from build123d import *

# Parameters (mm, degrees)
SKETCH1_W           = 137
SKETCH1_H           = 60
BOSS_EXTRUDE1_DEPTH = 6.5
SKETCH2_W           = 101
SKETCH2_H           = 55.5
CUT_EXTRUDE1_DEPTH  = 1.65
SKETCH3_W           = 87.3
SKETCH3_H           = 55.5
CUT_EXTRUDE2_DEPTH  = 4.1
SKETCH4_W           = 75.4
SKETCH4_H           = 51.7
CUT_EXTRUDE3_DEPTH  = 1.75
FILLET1_R           = 1
SKETCH6_W           = 7.15
SKETCH6_H           = 8
SKETCH6_W_2         = 6.55
CUT_EXTRUDE4_DEPTH  = 2.5
FILLET2_R           = 3
CHAMFER1_SIZE       = 0.5
SKETCH7_W           = 21
SKETCH7_H           = 52.453625608
CUT_EXTRUDE5_DEPTH  = 7.5
FILLET3_R           = 3
FILLET5_R           = 2
CHAMFER3_SIZE       = 1
FILLET6_R           = 1.5
FILLET7_R           = 1


with BuildPart() as part:
    # Sketch1 → Boss-Extrude1 (new body)
    with BuildSketch(Plane(origin=(0, 0, 0), x_dir=(1, 0, 0), z_dir=(0, 1, 0))):
        Rectangle(SKETCH1_W, SKETCH1_H)
    extrude(amount=BOSS_EXTRUDE1_DEPTH)

    # Sketch2 → Cut-Extrude1 (cut)
    with BuildSketch(Plane(origin=(0, 6.5, 0), x_dir=(1, 0, 0), z_dir=(0, 1, 0))):
        with Locations((14, 0)):
            Rectangle(SKETCH2_W, SKETCH2_H)
    extrude(amount=-CUT_EXTRUDE1_DEPTH, mode=Mode.SUBTRACT)

    # Sketch3 → Cut-Extrude2 (cut)
    with BuildSketch(Plane(origin=(0, 4.85, 0), x_dir=(1, 0, 0), z_dir=(0, 1, 0))):
        with Locations((13.7, 0)):
            Rectangle(SKETCH3_W, SKETCH3_H)
    extrude(amount=-CUT_EXTRUDE2_DEPTH, mode=Mode.SUBTRACT)

    # Sketch4 → Cut-Extrude3 (cut, through all)
    with BuildSketch(Plane(origin=(0, 0.75, 0), x_dir=(1, 0, 0), z_dir=(0, 1, 0))):
        with Locations((17.1, 0)):
            Rectangle(SKETCH4_W, SKETCH4_H)
    extrude(amount=-CUT_EXTRUDE3_DEPTH, mode=Mode.SUBTRACT)

    # Fillet1
    fillet1_edges = [part.edges().sort_by_distance(p)[0] for p in [
        (54.8, 0.375, -25.85),
        (54.8, 0.375, 25.85),
        (-20.6, 0.375, 25.85),
        (-20.6, 0.375, -25.85),
    ]]
    fillet(fillet1_edges, radius=FILLET1_R)

    # Sketch6 → Cut-Extrude4 (cut)
    with BuildSketch(Plane(origin=(0, 4.85, 0), x_dir=(1, 0, 0), z_dir=(0, 1, 0))):
        with Locations((60.925, -23.75)):
            Rectangle(SKETCH6_W, SKETCH6_H)
        with Locations((60.925, 23.75)):
            Rectangle(SKETCH6_W, SKETCH6_H)
        with Locations((-33.225, 23.75)):
            Rectangle(SKETCH6_W_2, SKETCH6_H)
        with Locations((-33.225, -23.75)):
            Rectangle(SKETCH6_W_2, SKETCH6_H)
    extrude(amount=-CUT_EXTRUDE4_DEPTH, mode=Mode.SUBTRACT)

    # Fillet2
    fillet2_edges = [part.edges().sort_by_distance(p)[0] for p in [
        (-29.95, 3.6, 19.75),
        (-29.95, 3.6, -19.75),
        (57.35, 3.6, -19.75),
        (57.35, 3.6, 19.75),
    ]]
    fillet(fillet2_edges, radius=FILLET2_R)

    # Chamfer1
    chamfer1_edges = [part.edges().sort_by_distance(p)[0] for p in [
        (17.1, 0, -25.85),
        (54.8, 0, 0),
        (17.1, 0, 25.85),
        (-20.6, 0, 0),
        (54.507106781, 0, -25.557106781),
        (54.507106781, 0, 25.557106781),
        (-20.307106781, 0, 25.557106781),
        (-20.307106781, 0, -25.557106781),
    ]]
    chamfer(chamfer1_edges, length=CHAMFER1_SIZE)

    # Sketch7 → Cut-Extrude5 (cut, through all)
    with BuildSketch(Plane(origin=(0, 6.5, 0), x_dir=(1, 0, 0), z_dir=(0, 1, 0))):
        with Locations((-52.5, 0)):
            Rectangle(SKETCH7_W, SKETCH7_H)
    extrude(amount=-CUT_EXTRUDE5_DEPTH, mode=Mode.SUBTRACT)

    # Fillet3
    fillet3_edges = [part.edges().sort_by_distance(p)[0] for p in [
        (-42, 3.25, -26.226812804),
        (-42, 3.25, 26.226812804),
        (-63, 3.25, 26.226812804),
        (-63, 3.25, -26.226812804),
    ]]
    fillet(fillet3_edges, radius=FILLET3_R)

    # Fillet5
    fillet5_edges = [part.edges().sort_by_distance(p)[0] for p in [
        (-34.725, 4.85, -19.75),
        (62.425, 4.85, 19.75),
        (62.425, 4.85, -19.75),
        (57.35, 4.85, 0),
        (58.228679656, 4.85, 18.871320344),
        (58.228679656, 4.85, -18.871320344),
        (-34.725, 4.85, 19.75),
        (-29.95, 4.85, 0),
        (-30.828679656, 4.85, -18.871320344),
        (-30.828679656, 4.85, 18.871320344),
    ]]
    fillet(fillet5_edges, radius=FILLET5_R)

    # Chamfer3
    chamfer3_edges = [part.edges().sort_by_distance(p)[0] for p in [
        (-29.95, 2.35, 22.25),
        (-29.95, 2.35, -22.25),
        (57.35, 2.35, -22.25),
        (57.35, 2.35, 22.25),
    ]]
    chamfer(chamfer3_edges, length=CHAMFER3_SIZE)

    # Fillet6
    fillet6_edges = [part.edges().sort_by_distance(p)[0] for p in [
        (68.5, 3.25, 30),
        (-68.5, 3.25, 30),
        (-68.5, 3.25, -30),
        (68.5, 3.25, -30),
    ]]
    fillet(fillet6_edges, radius=FILLET6_R)

    # Fillet7
    fillet7_edges = [part.edges().sort_by_distance(p)[0] for p in [
        (-42, 0, 0),
        (-52.5, 0, 26.226812804),
        (-63, 0, 0),
        (-52.5, 0, -26.226812804),
        (-42.878679656, 0, 25.348133148),
        (-62.121320344, 0, 25.348133148),
        (-62.121320344, 0, -25.348133148),
        (-42.878679656, 0, -25.348133148),
        (68.5, 0, 0),
        (0, 0, 30),
        (-68.5, 0, 0),
        (0, 0, -30),
        (68.060660172, 0, -29.560660172),
        (-68.060660172, 0, -29.560660172),
        (-68.060660172, 0, 29.560660172),
        (68.060660172, 0, 29.560660172),
    ]]
    fillet(fillet7_edges, radius=FILLET7_R)


solid = part.part
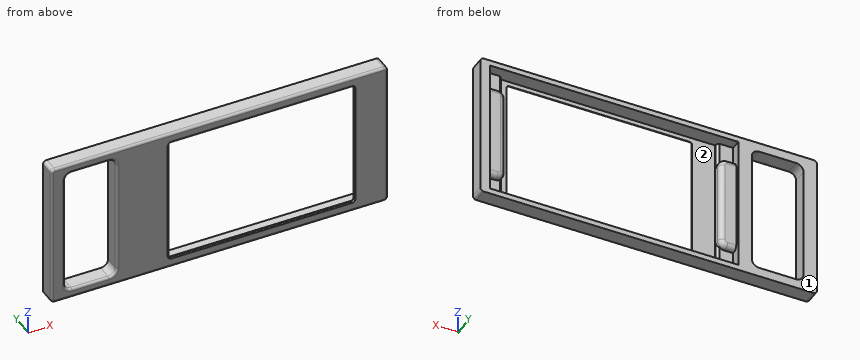
CAD build for the part. Positions are in the model's coordinates, mm. Face numbers are marked on the shaded views. Round coordinates to 2 decimals unless told otherwise and drop trailing zeros. Order: outer loops, then holes, each group sorted by start corner. A loop starts at its lowest first (then second) coordinate and runs counter-clockwise, first axis right, second up. Notation, with made-up numbers: (79.25, 9) -> (83.25, 9) arc R17 cw to (83.25, 14) -> close; hole circle Ø3 at (-9, 36). An arc over 180 degrees is marked (long way). Write item = value, one per line. Start each with the question number.
(1) Probe line 1 (X direction, y = 2.5, z = 12); line 2 (X direction, y = 6, z = -1.5); line 3 (Z direction, x = 38, y = 1.5). List the from-to ranges inside material, lowest first. Write a range as [from, to].
(2) Pin check, flat tips, straight feed: P1, Ø3, axis at x = -34.5, z = -23.5, coming from the +Y side; P2, Ø1.5, axis at x = 61.5, z = -7.5, coming from the +Y side. Stop position of each tip, or through.
(3) Cut at B-B, the plane x = -13. List the corners of the cut face in (y, z), then the cut area to 3 significant figures.
(4) Cut at A-A, the plane z = -21. List the corners of the cut face in (x, y), then the cut area to 3 significant figures.
(5) Cut at C-C, the plane z = 9. List the corners of the cut face in (x, y), then the cut area to 3 significant figures.
(6) Pull direction Z, two halves, no side cores. Call the marked faces 1 and 2: released by +Z, released by -Z, zero draft, split by the parting line, or undercut.
Model answer:
q1.line_1 = [-68.5, -63], [-42, -29.95], [57.35, 68.5]
q1.line_2 = [-68.5, -63], [-42, -36.5], [64.5, 68.5]
q1.line_3 = [-30, -27.75], [27.75, 30]
q2.P1 = 2.35
q2.P2 = 4.85
q3.outline = (0, -29) arc R1 ccw to (1, -30) -> (6.5, -30) -> (6.5, -27.75) -> (0.75, -27.75) -> (0.75, -25.85) -> (0.5, -25.85) -> (0, -26.35) -> close; (0, 26.35) -> (0.5, 25.85) -> (0.75, 25.85) -> (0.75, 27.75) -> (6.5, 27.75) -> (6.5, 30) -> (1, 30) arc R1 ccw to (0, 29) -> close
q3.area = 31.4 mm2
q4.outline = (-68.5, 1) arc R1 ccw to (-67.5, 0) -> (-64, 0) arc R1 ccw to (-63, 1) -> (-63, 6.5) -> (-68.5, 6.5) -> close; (-42, 1) arc R1 ccw to (-41, 0) -> (-21.1, 0) -> (-20.6, 0.5) -> (-20.6, 0.75) -> (-29.95, 0.75) -> (-29.95, 1.35) -> (-30.95, 2.35) -> (-36.5, 2.35) -> (-36.5, 6.5) -> (-42, 6.5) -> close; (54.8, 0.5) -> (55.3, 0) -> (67.5, 0) arc R1 ccw to (68.5, 1) -> (68.5, 6.5) -> (64.5, 6.5) -> (64.5, 2.35) -> (58.35, 2.35) -> (57.35, 1.35) -> (57.35, 0.75) -> (54.8, 0.75) -> close
q4.area = 137 mm2
q5.outline = (-68.5, 1) arc R1 ccw to (-67.5, 0) -> (-64, 0) arc R1 ccw to (-63, 1) -> (-63, 6.5) -> (-68.5, 6.5) -> close; (-42, 1) arc R1 ccw to (-41, 0) -> (-21.1, 0) -> (-20.6, 0.5) -> (-20.6, 0.75) -> (-29.95, 0.75) -> (-29.95, 2.85) arc R2 ccw to (-31.95, 4.85) -> (-36.5, 4.85) -> (-36.5, 6.5) -> (-42, 6.5) -> close; (54.8, 0.5) -> (55.3, 0) -> (67.5, 0) arc R1 ccw to (68.5, 1) -> (68.5, 6.5) -> (64.5, 6.5) -> (64.5, 4.85) -> (59.35, 4.85) arc R2 ccw to (57.35, 2.85) -> (57.35, 0.75) -> (54.8, 0.75) -> close
q5.area = 170 mm2
q6.face_1 = zero draft
q6.face_2 = undercut
